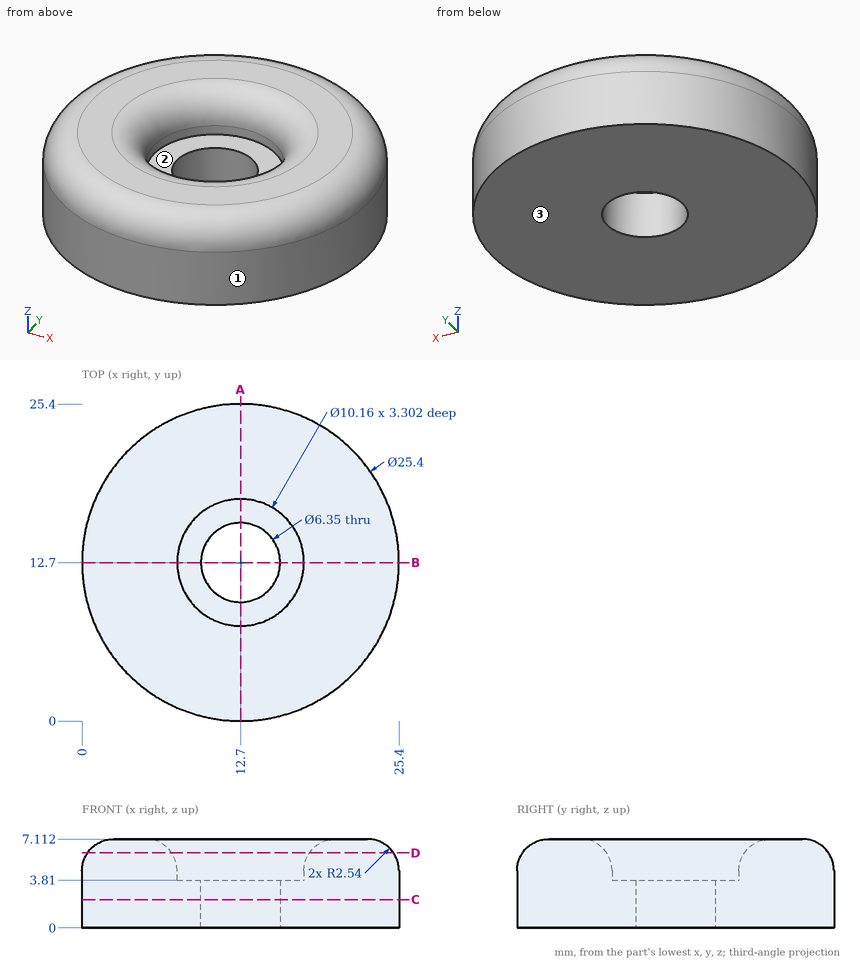
Drawing for the job (mm, zero at the part's lowest x, y, z). Coordinates: 2 decimals unless noted, no trailing zeros. Order: outer loops, then holes, each group sorted by start corner. A loop starts at its lowest first (then second) coordinate and runs counter-clockwise, first axis right, second up.
Item 1: Band-saw the part on C-C on z = 2.25. List the corners of the cut face in (x, y) (3 decimals), plus the area to 3 significant figures.
Check sheet entries:
outline: circle Ø25.4 at (12.7, 12.7); hole circle Ø6.35 at (12.7, 12.7)
area: 475 mm2
Item 2: Band-saw the part on D-D on z = 6. List the corners of the cut face in (x, y).
Check sheet entries:
outline: circle Ø24.52 at (12.7, 12.7); hole circle Ø11.04 at (12.7, 12.7)
Item 3: Drill centre lines: L1, parallel to Y at x = 12.7, z = 1.3 (3 decimals); L2, parallel to X at y = 9, z = 4.5; L3, parallel to Y at x = 9.75, z = 6.5. Where is each one in solid material? Low to high.
Check sheet entries:
L1: y = 0 to 9.525, 15.875 to 25.4
L2: x = 0.55 to 9.22, 16.18 to 24.85
L3: y = 1.26 to 7.51, 17.89 to 24.14
Item 4: Pin check, flat tips, straight feed: pin 1 Ø7.5 at (x, y) = (12.7, 12.7) entering from +Z; pin 2 Ø4 at (y, z) = (9, 2.5) entering from +X. Stop position of each tip, or through.
Check sheet entries:
pin 1: stops at z = 3.81
pin 2: stops at x = 25.29
Item 5: Band-saw the part on A-A on x = 12.7. List the corners of the cut face in (y, z) (3 decimals).
Check sheet entries:
outline: (0, 0) - (9.525, 0) - (9.525, 3.81) - (7.62, 3.81) - (7.62, 4.572) arc R2.54 ccw to (5.08, 7.112) - (2.54, 7.112) arc R2.54 ccw to (0, 4.572) - close; (15.875, 0) - (25.4, 0) - (25.4, 4.572) arc R2.54 ccw to (22.86, 7.112) - (20.32, 7.112) arc R2.54 ccw to (17.78, 4.572) - (17.78, 3.81) - (15.875, 3.81) - close
Item 6: Two-plate mould, pull along X, no slides. Class the marked faces 1, 2 and 3: +X half, -X half, draft (parallel to the pull), parting line (faces both ways), or undercut.
Check sheet entries:
face 1: parting line
face 2: undercut
face 3: draft
